from build123d import *

# Parameters (mm, degrees)
SKETCH_1_W          = 40
SKETCH_1_H          = 40
EXTRUDE_1_DEPTH     = 5
SKETCH_2_W          = 40
SKETCH_2_H          = 5
EXTRUDE_2_DEPTH     = 35
SKETCH_3_W          = 40
SKETCH_3_H          = 10
EXTRUDE_3_DEPTH     = 5
EXTRUDE_4_DEPTH     = 5
SKETCH_5_R          = 2.25
CUT_EXTRUDE_1_DEPTH = 20
CUT_EXTRUDE_2_DEPTH = 40
SKETCH_7_W          = 40
SKETCH_7_H          = 19
CUT_EXTRUDE_3_DEPTH = 20
SKETCH_8_W          = 40
SKETCH_8_H          = 1.5
CUT_EXTRUDE_4_DEPTH = 16
SKETCH_9_R          = 1.2
CUT_EXTRUDE_5_DEPTH = 20


with BuildPart() as part:
    # 草图1 → 凸台-拉伸1 (new body)
    with BuildSketch(Plane(origin=(0, 0, 0), x_dir=(1, 0, 0), z_dir=(0, 1, 0))):
        Rectangle(SKETCH_1_W, SKETCH_1_H)
    extrude(amount=EXTRUDE_1_DEPTH)

    # 草图2 → 凸台-拉伸2 (add)
    with BuildSketch(Plane(origin=(0, 5, 0), x_dir=(1, 0, 0), z_dir=(0, 1, 0))):
        with Locations((0, 1.5)):
            Rectangle(SKETCH_2_W, SKETCH_2_H)
    extrude(amount=EXTRUDE_2_DEPTH)

    # 草图3 → 凸台-拉伸3 (add)
    with BuildSketch(Plane.XZ):
        with Locations((0, 15)):
            Rectangle(SKETCH_3_W, SKETCH_3_H)
    extrude(amount=EXTRUDE_3_DEPTH)

    # 草图4 → 凸台-拉伸4 (add)
    with BuildSketch(Plane.XZ.offset(5)):
        Polygon((-20, 10), (-20, -20), (20, -20), (20, 10), (20, 20), (-20, 20), align=None)
    extrude(amount=EXTRUDE_4_DEPTH)

    # 草图5 → 切除-拉伸1 (cut)
    with BuildSketch(Plane(origin=(0, 5, 0), x_dir=(1, 0, 0), z_dir=(0, 1, 0))):
        with Locations(Location((-14.795139738, 14, 0), (0, 0, 90))):
            Circle(SKETCH_5_R)
        with Locations(Location((14.795139738, 14, 0), (0, 0, 90))):
            Circle(SKETCH_5_R)
    extrude(amount=-CUT_EXTRUDE_1_DEPTH, mode=Mode.SUBTRACT)

    # 草图6 → 切除-拉伸2 (cut)
    with BuildSketch(Plane.ZY.offset(20)):
        Polygon((10, 0), (20, 0), (20, -10), (-20, -10), (-20, -5), (10, -5), align=None)
    extrude(amount=-CUT_EXTRUDE_2_DEPTH, mode=Mode.SUBTRACT)

    # 草图7 → 切除-拉伸3 (cut)
    with BuildSketch(Plane(origin=(0, 5, 0), x_dir=(1, 0, 0), z_dir=(0, 1, 0))):
        with Locations((0, -10.5)):
            Rectangle(SKETCH_7_W, SKETCH_7_H)
    extrude(amount=-CUT_EXTRUDE_3_DEPTH, mode=Mode.SUBTRACT)

    # 草图8 → 切除-拉伸4 (cut)
    with BuildSketch(Plane(origin=(0, 0, -20), x_dir=(-1, 0, 0), z_dir=(0, 0, -1))):
        with Locations((0, 4.25)):
            Rectangle(SKETCH_8_W, SKETCH_8_H)
    extrude(amount=-CUT_EXTRUDE_4_DEPTH, mode=Mode.SUBTRACT)

    # 草图9 → 切除-拉伸5 (cut)
    with BuildSketch(Plane.XY.offset(1)):
        with Locations((13.5, 6.5)):
            Circle(SKETCH_9_R)
        with Locations((-13.5, 6.5)):
            Circle(SKETCH_9_R)
        with Locations((-13.5, 33.5)):
            Circle(SKETCH_9_R)
        with Locations((13.5, 33.5)):
            Circle(SKETCH_9_R)
    extrude(amount=-CUT_EXTRUDE_5_DEPTH, mode=Mode.SUBTRACT)


solid = part.part
Work out the finished part from the listing and answer in its coordinate system (mm). A direction names the side the tool comes from. Round coordinates to 2 decimals unless told otherwise and drop trailing zeros. Loops run counter-clockwise (first coordinate to the right, second up) from the corner with the lowest first, then second, coordinate; pieces in that order, holes last. Notation, with made-up numbers: (-15, 25) -> (18, 25) arc R10 cw to (18, 40) -> close; hole circle Ø3 at (67.5, -11). An arc over 180 degrees is marked (long way). Use one line per item in the form item = value.
(1) For a pull along Y with two mould halves and no side action, classify faces 1 (the cylindrical face through (13.34, 34.69, -1.46)), 2 (the cylindrical face through (-12.8, 1.77, -15.04)), 3 (the flat face through (0, 0, -10)) as released by +Y, released by -Y, zero draft, split by the parting line, or undercut.
Answer list:
face_1 = undercut
face_2 = zero draft
face_3 = released by -Y
(2) Straight lines are drawn through the part: line 1 (Y direction, x = 13.5, z = -1.65); line 2 (Z direction, x = -15.5, y = 16); line 3 (Y direction, x = 3, z = -5.75). For each, find the intervals that lie inside material, in ascending order.
Answer list:
line_1 = 0 to 5.3, 7.7 to 32.3, 34.7 to 40
line_2 = -4 to 1
line_3 = 0 to 3.5
(3) Find section C-C on x = 13.5. Give the vertices of the cut face in (y, z).
Answer list:
outline = (0, -20) -> (3.5, -20) -> (3.5, -15.84) -> (0, -15.84) -> close; (0, -12.16) -> (3.5, -12.16) -> (3.5, -4) -> (5.3, -4) -> (5.3, 1) -> (0, 1) -> close; (7.7, -4) -> (32.3, -4) -> (32.3, 1) -> (7.7, 1) -> close; (34.7, -4) -> (40, -4) -> (40, 1) -> (34.7, 1) -> close
(4) Find section A-A on y = 6.5. Give the vertices of the cut face in (x, z).
Answer list:
outline = (-20, -4) -> (-14.7, -4) -> (-14.7, 1) -> (-20, 1) -> close; (-12.3, -4) -> (12.3, -4) -> (12.3, 1) -> (-12.3, 1) -> close; (14.7, -4) -> (20, -4) -> (20, 1) -> (14.7, 1) -> close
(5) Find section D-D on x = 8. Give the vertices of the cut face in (y, z), then the cut area to 3 significant figures.
Answer list:
outline = (0, -20) -> (3.5, -20) -> (3.5, -4) -> (40, -4) -> (40, 1) -> (0, 1) -> close
area = 256 mm2
(6) Flat-ended cylindrical pins translate along their axes: P1, Ø6, axis at x = -10, y = 8.5, coming from the -Z side; P2, Ø1, axis at x = 4, z = -14, coming from the +Y side; P3, Ø1.9, axis at x = -13.5, y = 6.5, coming from the -Z side. Find the tip coordinate at first contact, or state that the pin passes through.
Answer list:
P1 = -4
P2 = 3.5
P3 = through
(7) Find section B-B on z = -14. Give the vertices of the cut face in (x, y), then the cut area to 4 significant figures.
Answer list:
outline = (-20, 0) -> (-17.05, 0) -> (-17.05, 3.5) -> (-20, 3.5) -> close; (-12.55, 0) -> (12.55, 0) -> (12.55, 3.5) -> (-12.55, 3.5) -> close; (17.05, 0) -> (20, 0) -> (20, 3.5) -> (17.05, 3.5) -> close
area = 108.5 mm2
(8) A tool of negligible diameter and unlimited length cuts with its end or side. For faces 4 (the flat face through (0, 21, -4)), 5 (the cylindrical face through (16.79, 1.77, -15.04)), from which of +Z, -Z, +X, -X, +Y, -Y can it reach the whole face along a straight path? Write none if from no direction.
Answer list:
face_4 = -Z, +X, -X, +Y
face_5 = +Y, -Y
